Could you check a few things on this model? Use its own coordinates, in mm. A direction names the side the tool comes from. Coordinates: 2 decimals unless noted, no trailing zeros. Write each loop counter-clockwise with the first axis right and the second up, starting at its lowest first coordinate (ties: lowest second). Pieces come first, ordered by that corner, then holes.
```python
from build123d import *

# Parameters (mm, degrees)
F0_W     = 545
F0_H     = 465
F1_DEPTH = 575
F2_W     = 120
F2_H     = 12
F3_DEPTH = 10
F4_W     = 136.365123
F4_H     = 465
F5_DEPTH = 10


with BuildPart() as f1:
    # F0 (on Front) → F1 (new body)
    with BuildSketch(Plane.XZ):
        Rectangle(F0_W, F0_H)
    extrude(amount=-F1_DEPTH)

    # F2 (on face) → F3 (join)
    with BuildSketch(Plane(origin=(0, 575, 0), x_dir=(-1, 0, 0), z_dir=(0, 1, 0))):
        with Locations((0, 160.409869)):
            Rectangle(F2_W, F2_H)
    extrude(amount=F3_DEPTH)

    # F4 (on face) → F5 (join)
    with BuildSketch(Plane.XZ):
        with Locations((188.826646, 0)):
            Rectangle(F4_W, F4_H)
    extrude(amount=F5_DEPTH)


solid = f1.part
```
1. I want a section at D-D on x = 160. Please give me the cut outline in (y, z), plus the area to 3 significant figures.
Verdict:
outline: (-10, -232.5) - (575, -232.5) - (575, 232.5) - (-10, 232.5) - close
area: 272,000 mm2
2. On a 3-axis mill with a long thin cutter (end or side, diameter ignored), from which of +Z, -Z, +X, -X, +Y, -Y can I reach the whole of each face in a straight line? I mean faces 1 (the face through (265, 0, 3)), 2 (the face through (-79, 0, 3)), 3 (the face through (272.5, 283, -3)). Say none if no direction works.
Verdict:
face 1: +Z, -Z, +X, -Y
face 2: +Z, -Z, -X, -Y
face 3: +Z, -Z, +X, +Y, -Y
3. Please list where these lines run through material, in increasing order: line 1 along Y through (x, z) = (-195, -209); line 2 along Y through (x, z) = (129.5, 107.5).
Verdict:
line 1: y = 0 to 575
line 2: y = -10 to 575
4. I want a section at B-B on x = 39. Please give me the cut outline in (y, z), plus the area to 3 significant figures.
Verdict:
outline: (0, -232.5) - (575, -232.5) - (575, 154.41) - (585, 154.41) - (585, 166.41) - (575, 166.41) - (575, 232.5) - (0, 232.5) - close
area: 267,000 mm2
5. I want a section at A-A on z = 31. Please give me the cut outline in (x, y).
Verdict:
outline: (-272.5, 0) - (120.64, 0) - (120.64, -10) - (257.01, -10) - (257.01, 0) - (272.5, 0) - (272.5, 575) - (-272.5, 575) - close
6. I want a section at C-C on x = -81.5. Please give me the cut outline in (y, z).
Verdict:
outline: (0, -232.5) - (575, -232.5) - (575, 232.5) - (0, 232.5) - close
7. For pin 1 (5 mm diameter, centred on x = 216.5, z = 172.5, fed in from +Y); pin 2 (8 mm diameter, centred on y = -5.5, z = 17, fed in from +X); pin 3 (5 mm diameter, centred on x = -10, z = 92.5, fed in from -Y), each with a flat end and sliding along its axis, tell me the tip position at first contact or that it passes through.
Verdict:
pin 1: stops at y = 575
pin 2: stops at x = 257.01
pin 3: stops at y = 0
